```python
from build123d import *

# Parameters (mm, degrees)
F0_W     = 86.436784
F0_H     = 80
F1_DEPTH = 80
F2_R     = 15
F3_DEPTH = 80.001
F4_R     = 5


with BuildPart() as f1:
    # F0 (on Top) → F1 (new body)
    with BuildSketch(Plane.XY):
        Rectangle(F0_W, F0_H)
    extrude(amount=F1_DEPTH)

    # F2 (on face) → F3 (cut, through all)
    with BuildSketch(Plane.XY.offset(80)):
        Circle(F2_R)
    extrude(amount=-F3_DEPTH, mode=Mode.SUBTRACT)

    # F4
    f4_edges = [f1.edges().sort_by_distance(p)[0] for p in [
        (-43.218392, -40, 40),
        (-43.218392, 0, 0),
        (-43.218392, 40, 40),
        (0, -40, 0),
        (0, 40, 0),
        (43.218392, 0, 0),
        (0, 40, 80),
        (-43.218392, 0, 80),
        (0, -40, 80),
        (43.218392, 0, 80),
        (-15, 0, 80),
        (-15, 0, 0),
    ]]
    fillet(f4_edges, radius=F4_R)


solid = f1.part
```
Can you work these out from the model? Positions are in its coordinate system, mm. Coordinates: 2 decimals unless noted, no trailing zeros. Write each loop counter-clockwise with the first axis right and the second up, starting at its lowest first coordinate (ties: lowest second). Pieces come first, ordered by that corner, then holes. Notation, with made-up numbers: M 1.5,59.25 L 35.5,59.25 A20 ccw 35.5,74.25 Z; hole C 19,-37 d6. An arc over 180 degrees is marked long. Write item = value, one per line. Start each with the question number.
Q1. I'm going to push a flat-ended pin straight in: pin 1 (1 mm diameter, centred on x = -18, y = 3, fed in from -Z). Where does the tip first touch, or does it pass through?
Q2. If we section it at B-B, the plane z = 57: Write out the boundary of the cut face in (x, y).
Q3. If we section it at A-A, the plane y = 0: Write out the boundary of the cut face in (x, z), then the cut area to 3 significant figures.
Q4. If we section it at C-C, the plane x = 0: Write out the boundary of the cut face in (y, z), then the cut area to 3 significant figures.
Q5. If I drill on L1, parallel to Y at x = 0, z = 47.5; L2, parallel to X at y = 35.5, z = 71; L3, parallel to Y at x = 10, z = 7, over which ranges is the centre line in solid material (lowest first)? Write a range as [from, to].
Q6. Thinking about a two-plate mould opening in X: for faces 1 (the face through (3, 39, 2)), 2 (the face through (-14.985, 0.66, 40.49)), 3 (the face through (-41.79, 38.5, 40.49)), which applies, released by +X, released by -X, zero draft, split by the parting line, or undercut?
Check sheet entries:
q1.pin_1 = 0.16
q2.outline = M -43.22,-35 A5 ccw -38.22,-40 L 43.22,-40 L 43.22,40 L -38.22,40 A5 ccw -43.22,35 Z; hole C 0,0 d30
q3.outline = M -43.22,5 A5 ccw -38.22,0 L -20,0 A5 ccw -15,5 L -15,75 A5 ccw -20,80 L -38.22,80 A5 ccw -43.22,75 Z; M 15,5 A5 ccw 20,0 L 38.22,0 A5 ccw 43.22,5 L 43.22,75 A5 ccw 38.22,80 L 20,80 A5 ccw 15,75 Z
q3.area = 4,470 mm²
q4.outline = M -40,5 A5 ccw -35,0 L -20,0 A5 ccw -15,5 L -15,75 A5 ccw -20,80 L -35,80 A5 ccw -40,75 Z; M 15,5 A5 ccw 20,0 L 35,0 A5 ccw 40,5 L 40,75 A5 ccw 35,80 L 20,80 A5 ccw 15,75 Z
q4.area = 3,960 mm²
q5.L1 = [-40, -15], [15, 40]
q5.L2 = [-43.19, 43.22]
q5.L3 = [-40, -11.18], [11.18, 40]
q6.face_1 = zero draft
q6.face_2 = undercut
q6.face_3 = released by -X
